Geometry: final body of the model. Coordinates: model frame, mm. Face numbers are marked on the shaded views. A direction names the side the tool comes from. Give positions to 0.01 mm unless a question says otherwise; leave off trailing zeros. Order: outer loops, then holes, each group sorted by start corner. A loop starts at its lowest first (then second) coordinate and runs counter-clockwise, first axis right, second up. Notation, with made-up numbers: (40, 46.25) -> (55, 46.25) arc R34 cw to (55, 83.25) -> close; hole circle Ø3 at (63.25, 80.25). An arc over 180 degrees is marked (long way). Write item = value, one per line.
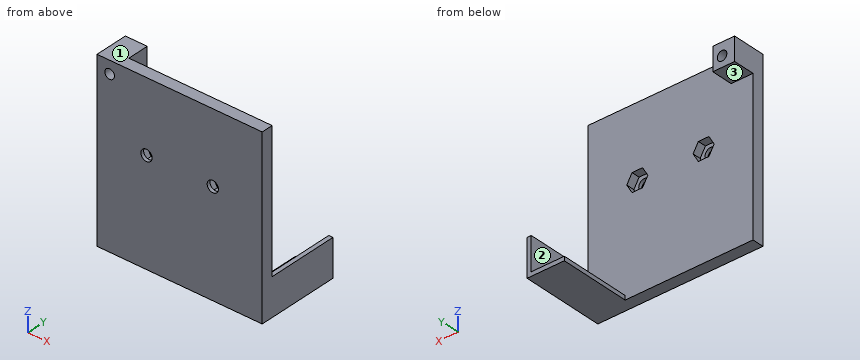
```python
from build123d import *

# Parameters (mm, degrees)
BOSS_EXTRUDE1_DEPTH = 3.5
BOSS_EXTRUDE2_DEPTH = 25
SKETCH1_5_W         = 6.602272727
SKETCH1_5_H         = 7
BOSS_EXTRUDE3_DEPTH = 10
SKETCH3_R           = 1.45
CUT_EXTRUDE1_DEPTH  = 40.267925843
SKETCH4_R           = 1.7
CUT_EXTRUDE2_DEPTH  = 43.18080132
SKETCH4_3_R         = 1.7
CUT_EXTRUDE3_DEPTH  = 2.5


with BuildPart() as part:
    # Sketch1 → Boss-Extrude1 (new body)
    with BuildSketch(Plane(origin=(0, 0, 0), x_dir=(1, 0, 0), z_dir=(0, 1, 0))):
        Polygon((13.65, 25.15), (13.65, 26.4), (-24.9, 26.4), (-24.9, -19.4), (-18.297727273, -19.4), (-18.297727273, -26.4), (24.9, -26.4), (24.9, 15.15), (23.65, 15.15), (23.65, 25.15), align=None)
    extrude(amount=BOSS_EXTRUDE1_DEPTH)

    # Sketch1_4 → Boss-Extrude2 (add)
    with BuildSketch(Plane(origin=(0, 0, 0), x_dir=(1, 0, 0), z_dir=(0, 1, 0))):
        Polygon((24.9, 26.4), (13.65, 26.4), (13.65, 25.15), (23.65, 25.15), (23.65, 15.15), (24.9, 15.15), align=None)
    extrude(amount=BOSS_EXTRUDE2_DEPTH)

    # Sketch1_5 → Boss-Extrude3 (add)
    with BuildSketch(Plane(origin=(0, 0, 0), x_dir=(1, 0, 0), z_dir=(0, 1, 0))):
        with Locations((-21.598863636, -22.9)):
            Rectangle(SKETCH1_5_W, SKETCH1_5_H)
    extrude(amount=BOSS_EXTRUDE3_DEPTH)

    # Sketch3 → Cut-Extrude1 (cut, through all)
    with BuildSketch(Plane(origin=(0, 10, 0), x_dir=(1, 0, 0), z_dir=(0, 1, 0))):
        with Locations(Location((-21.1, -22.6, 0), (0, 0, 270))):
            Circle(SKETCH3_R)
    extrude(amount=-CUT_EXTRUDE1_DEPTH, mode=Mode.SUBTRACT)

    # Sketch4 → Cut-Extrude2 (cut, through all)
    with BuildSketch(Plane(origin=(0, 3.5, 0), x_dir=(1, 0, 0), z_dir=(0, 1, 0))):
        with Locations(Location((-10, -5, 0), (0, 0, 270))):
            Circle(SKETCH4_R)
        with Locations(Location((10, -5, 0), (0, 0, 270))):
            Circle(SKETCH4_R)
    extrude(amount=-CUT_EXTRUDE2_DEPTH, mode=Mode.SUBTRACT)

    # Sketch4_3 → Cut-Extrude3 (cut)
    # profile 1 of 2: a face of its own
    with BuildSketch(Plane(origin=(0, 3.5, 0), x_dir=(1, 0, 0), z_dir=(0, 1, 0))):
        Polygon((-6.824573519, -5), (-8.41228676, -2.25), (-11.58771324, -2.25), (-13.175426481, -5), (-11.58771324, -7.75), (-8.41228676, -7.75), align=None)
        with Locations(Location((-10, -5, 0), (0, 0, 270))):
            Circle(SKETCH4_3_R, mode=Mode.SUBTRACT)
    # profile 2 of 2: a face of its own
    with BuildSketch(Plane(origin=(0, 3.5, 0), x_dir=(1, 0, 0), z_dir=(0, 1, 0))):
        Polygon((13.175426481, -5), (11.58771324, -2.25), (8.41228676, -2.25), (6.824573519, -5), (8.41228676, -7.75), (11.58771324, -7.75), align=None)
        with Locations(Location((10, -5, 0), (0, 0, 270))):
            Circle(SKETCH4_3_R, mode=Mode.SUBTRACT)
    extrude(amount=-CUT_EXTRUDE3_DEPTH, mode=Mode.SUBTRACT)


solid = part.part
```
1) Section query B-B (z = 22.6). Output: boundary loops of the cut face in (x, y).
Check sheet entries:
outline = (-24.9, 0) -> (-22.55, 0) -> (-22.55, 10) -> (-24.9, 10) -> close; (-19.65, 0) -> (24.9, 0) -> (24.9, 3.5) -> (-18.3, 3.5) -> (-18.3, 10) -> (-19.65, 10) -> close
2) Section query A-A (y = 5.5). Output: boundary loops of the cut face in (x, z), plus the area to 3 significant figures.
Check sheet entries:
outline = (-24.9, 19.4) -> (-18.3, 19.4) -> (-18.3, 26.4) -> (-24.9, 26.4) -> close; (13.65, -26.4) -> (24.9, -26.4) -> (24.9, -15.15) -> (23.65, -15.15) -> (23.65, -25.15) -> (13.65, -25.15) -> close; hole circle Ø2.9 at (-21.1, 22.6)
area = 66.2 mm²
3) Section query D-D (y = 22.5). Output: boundary loops of the cut face in (x, z).
Check sheet entries:
outline = (13.65, -26.4) -> (24.9, -26.4) -> (24.9, -15.15) -> (23.65, -15.15) -> (23.65, -25.15) -> (13.65, -25.15) -> close
4) First-contact query: P1, Ø3, axis at x = 16.5, y = 11, coming from the +Z side; P2, Ø6, axis at x = 10.5, z = 6.5, coming from the +Y side; P3, Ø2, axis at y = 6, z = 21.5, coming from the +X side. Flat tips, straight axial feed; report the tip coordinate or a pass-through.
Check sheet entries:
P1 = -25.15
P2 = 3.5
P3 = -18.3
5) Reachability of the marked faces 1, 2 and 3 from +Z, -Z, +X, -X, +Y, -Y: full face, straight path, thin tool, end or side. Return the list, or none.
Check sheet entries:
face_1 = +Z, +X, -X, +Y, -Y
face_2 = +Z, -X, +Y
face_3 = -Z, +X, -X, +Y
6) Line query: line 1 (X direction, y = 0.45, z = 5); line 2 (X direction, y = 6, z = 22.6); line 3 (Z direction, x = 8.5, y = 2). Output: solid intervals per line, ascending. Write a range as from..to.
Check sheet entries:
line_1 = -24.9..-11.7, -8.3..8.3, 11.7..24.9
line_2 = -24.9..-22.55, -19.65..-18.3
line_3 = -26.4..2.25, 7.75..26.4
7) Section query C-C (x = -21.1). Output: boundary loops of the cut face in (y, z).
Check sheet entries:
outline = (0, -26.4) -> (3.5, -26.4) -> (3.5, 19.4) -> (10, 19.4) -> (10, 21.15) -> (0, 21.15) -> close; (0, 24.05) -> (10, 24.05) -> (10, 26.4) -> (0, 26.4) -> close
